Print and shaded views of the part. All mm, measured from the part's lowest x, y and z. A direction names the side the tool comes from. Round coordinates to 2 decimals unless told otherwise and drop trailing zeros. Write each loop counter-clockwise with the first axis right and the second up, starting at its lowest first coordinate (ties: lowest second). Pieces come first, ordered by that corner, then holes. Notation, with made-up numbers: M 51.5,-18.75 L 88.5,-18.75 A20 ccw 88.5,-2.75 Z; hole C -38,42.25 d4. An arc over 180 degrees is marked long. Write item = value, one per line. Start each with the question number.
Q1. Probe L1, parallel to Z at x = 26, y = 8; L2, parallel to Y at x = 26, z = 15; L3, parallel to Y at x = 26, z = 9. List the from-to ranges inside material, lowest first.
Q2. Band-saw the part on D-D on y = 3. Write the cut outline in (x, z), plus the area to 3 significant figures.
Q3. Band-saw the part on A-A on y = 26. Write the cut outline in (x, z).
Q4. Pull direction Y, two halves, no side cores. Call the marked faces 1, 2 and 3: released by +Y, released by -Y, zero draft, split by the parting line, or undercut.
Q5. Band-saw the part on B-B on x = 14.5. Write the cut outline in (y, z), plus the area to 3 significant figures.
Q6. Tool access for the marked faces 4 and 5: list every direction of +Z, -Z, +X, -X, +Y, -Y with a clear straight run to the whole face (end or side of a thin tool).
Q7. Band-saw the part on C-C on x = 26. Write the cut outline in (y, z), plus the area to 3 significant figures.
Q8. Drop flat-ended pins along their axis: P1, Ø8, axis at x = 40, z = 6.5, coming from the +Y side; P2, Ø9, axis at x = 26, z = 10, coming from the -Y side; P3, Ø1, axis at x = 9.5, z = 11, coming from the -Y side; P4, Ø10, axis at y = 20.5, z = 17.5, coming from the +X side. Give the stop position or say it passes through.
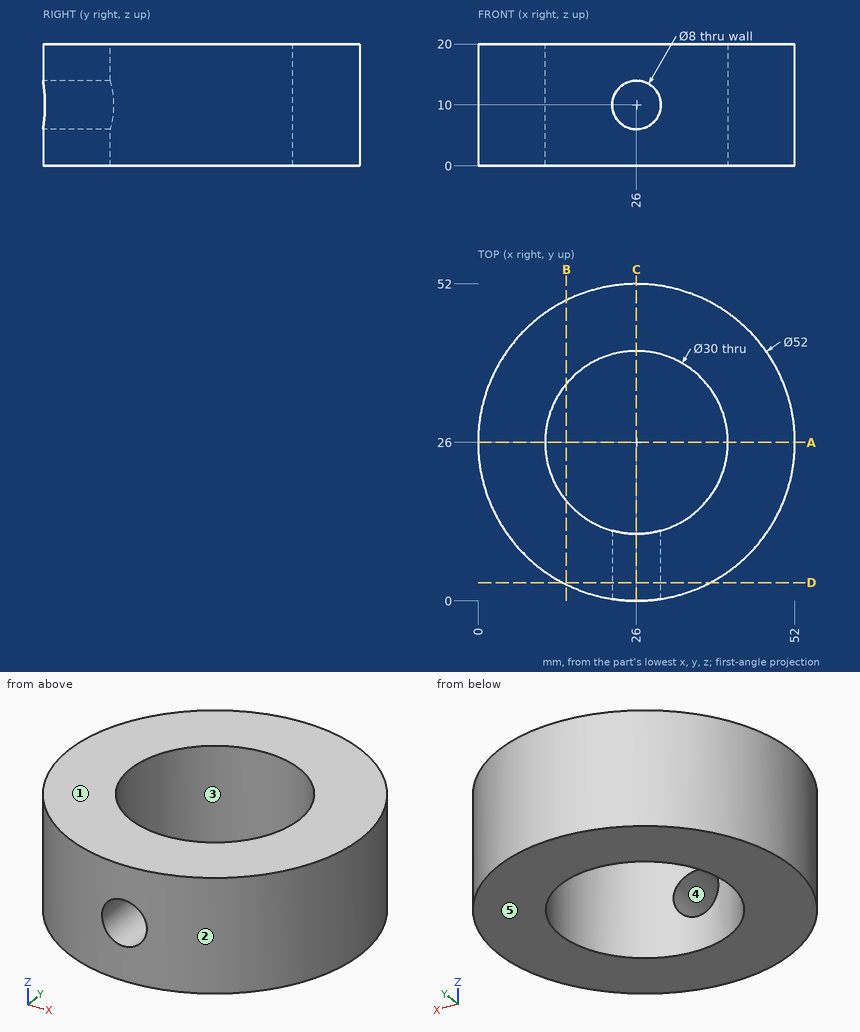
Conclusion:
q1.L1 = 0 to 6, 14 to 20
q1.L2 = 0 to 11, 41 to 52
q1.L3 = 41 to 52
q2.outline = M 13.88,0 L 38.12,0 L 38.12,20 L 13.88,20 Z; hole C 26,10 d8
q2.area = 435 mm^2
q3.outline = M 0,0 L 11,0 L 11,20 L 0,20 Z; M 41,0 L 52,0 L 52,20 L 41,20 Z
q4.face_1 = zero draft
q4.face_2 = split by the parting line
q4.face_3 = undercut
q5.outline = M 2.68,0 L 16.37,0 L 16.37,20 L 2.68,20 Z; M 35.63,0 L 49.32,0 L 49.32,20 L 35.63,20 Z
q5.area = 548 mm^2
q6.face_4 = -Y
q6.face_5 = -Z, +X, -X, +Y, -Y
q7.outline = M 0,0 L 11,0 L 11,6 L 0,6 Z; M 0,14 L 11,14 L 11,20 L 0,20 Z; M 41,0 L 52,0 L 52,20 L 41,20 Z
q7.area = 352 mm^2
q8.P1 = 50
q8.P2 = 0
q8.P3 = 5.51
q8.P4 = 52
